For this review, take the finished solid that the model builds, in its own axes (mm). A direction names the side the tool comes from. Give positions to 0.01 mm unless a question says otherwise; leave off trailing zeros. Order: outer loops, then holes, each group sorted by start corner. A loop starts at its lowest first (then second) coordinate and runs counter-clockwise, first axis right, second up. Notation, with made-up numbers: (40.25, -21) -> (93.25, -21) arc R20 ccw to (93.25, 2) -> close; hole circle Ø5 at (-22, -23). An arc over 180 degrees is marked (long way). Return JSON: item names as keys, results as strings. Group by question number.
1) Insertion check: P1, Ø3, axis at x = 2, z = 24, coming from the +Y side; P2, Ø4, axis at x = -14, y = -30.5, coming from the +Z side; P3, Ø12, axis at x = 31.5, y = -22.5, coming from the +Z side; P4, Ø2.5, axis at x = 0, y = 37.5, coming from the +Z side. Each pin has a flat end and moves straight along its axis. Give the tip position at first contact, or say it passes through.
2) For faces 4 (the face through (-14.6, 43.3, 30)), 5 (the face through (2.2, 37.6, 6)), 6 (the face through (-39.717, -19.697, 15.734)), 7 (the face through (42.604, 1.875, 14.434)), 8 (the face through (47, 0, 23)), list the 3-axis set-ups (+Z, -Z, +X, -X, +Y, -Y) from which the entire face can be reached by the end or side of a thin tool; tool diameter is ignored.
3) Add section C-C (x = 0). State how many separate pieces and enclosed holes the cut face has, then the cut area to 3 significant figures.
4) The part is to be moulded in two halves that separate along Y. For faces 1 (the face through (-22.38, -43.028, 14.79)), 2 (the face through (-1, 1, 0)), 3 (the face through (9, 1, 3)), say which applies: released by +Y, released by -Y, zero draft, split by the parting line, or undercut.
5) Add section B-B (y = 0). Give the boundary of the cut face in (x, z).
6) To check wall thickness, follow line 1 along Z through (x, y) = (-46.4, 0); line 2 along Y through (x, z) = (0, 16); line 3 along Y through (x, z) = (0, 6.5). State the ranges of each line that lie inside material, in increasing order.
7) Add section A-A (z = 4.5). Give the boundary of the cut face in (x, y).
from build123d import *

# Parameters (mm, degrees)
F2_R      = 2
F3_DEPTH  = 77.8
F4_R      = 5
F5_DEPTH  = 6
F6_R      = 2
F7_DEPTH  = 12.5
F8_DEPTH  = 12.5
F9_R      = 2
F10_DEPTH = 50
F11_R     = 17.5
F12_DEPTH = 25
F14_R     = 2
F15_DEPTH = 50
F17_R     = 2
F18_DEPTH = 50


with BuildPart() as f1:
    # F0 (on Front) → F1 (revolve)
    with BuildSketch(Plane.XZ):
        Polygon((-48.5, 0), (0, 0), (0, 3), (-45.5, 3), (-45.5, 11.58), (-45.5, 17.58), (-45.5, 30), (-48.5, 30), align=None)
        Polygon((-45.5, 17.58), (-45.5, 11.58), (-42.5, 14.58), (-42.5, 17.58), align=None)
    revolve(axis=Axis((0, 0, 1.5), (0, 0, -1)))

    # F2 (on Front) → F3 (cut, symmetric)
    with BuildSketch(Plane.XZ):
        with Locations((0, 21)):
            Circle(F2_R)
    extrude(amount=F3_DEPTH, both=True, mode=Mode.SUBTRACT)

    # F4 (on Top) → F5 (join)
    with BuildSketch(Plane.XY):
        with Locations((0, -37.5)):
            Circle(F4_R)
        with Locations((0, 37.5)):
            Circle(F4_R)
    extrude(amount=F5_DEPTH)

    # F6 (on face) → F7 (cut, symmetric)
    with BuildSketch(Plane.XY.offset(3)):
        with Locations((0, 37.5)):
            Circle(F6_R)
    extrude(amount=F7_DEPTH, both=True, mode=Mode.SUBTRACT)

    # F6 (on face) → F8 (cut, symmetric)
    with BuildSketch(Plane.XY.offset(3)):
        with Locations((0, -37.5)):
            Circle(F6_R)
    extrude(amount=F8_DEPTH, both=True, mode=Mode.SUBTRACT)

    # F9 (on Right) → F10 (cut, symmetric)
    with BuildSketch(Plane.YZ):
        with Locations((0, 21)):
            Circle(F9_R)
    extrude(amount=F10_DEPTH, both=True, mode=Mode.SUBTRACT)

    # F11 (on face) → F12 (cut, symmetric)
    with BuildSketch(Plane.XY.offset(3)):
        with Locations((-24, -12)):
            Circle(F11_R)
    extrude(amount=F12_DEPTH, both=True, mode=Mode.SUBTRACT)

    # F14 (on face) → F15 (cut, symmetric)
    with BuildSketch(Plane(origin=(0, 0, 0), x_dir=(0.707107, -0.707107, 0), z_dir=(-0.707107, -0.707107, 0))):
        with Locations((0, 21)):
            Circle(F14_R)
    extrude(amount=F15_DEPTH, both=True, mode=Mode.SUBTRACT)

    # F17 (on face) → F18 (cut, symmetric)
    with BuildSketch(Plane(origin=(0, 0, 0), x_dir=(-0.707107, -0.707107, 0), z_dir=(-0.707107, 0.707107, 0))):
        with Locations((0, 21)):
            Circle(F17_R)
    extrude(amount=F18_DEPTH, both=True, mode=Mode.SUBTRACT)


solid = f1.part
Evaluation:
{
 "1": {"P1": "y = 48.5", "P2": "z = 3", "P3": "z = 17.58", "P4": "through"},
 "2": {"face 4": "+Z, +X, -X, +Y, -Y", "face 5": "+Z", "face 6": "+Z, -Z", "face 7": "none", "face 8": "+X, -X"},
 "3": {"separate pieces": "5", "enclosed holes": "0", "area": "468 mm^2"},
 "4": {"face 1": "split by the parting line", "face 2": "zero draft", "face 3": "undercut"},
 "5": {"outline": "(-48.5, 0) -> (-36.74, 0) -> (-36.74, 3) -> (-45.5, 3) -> (-45.5, 11.58) -> (-42.5, 14.58) -> (-42.5, 17.58) -> (-45.5, 17.58) -> (-45.5, 19) -> (-48.5, 19) -> close; (-48.5, 23) -> (-45.5, 23) -> (-45.5, 30) -> (-48.5, 30) -> close; (-11.26, 0) -> (48.5, 0) -> (48.5, 19) -> (45.5, 19) -> (45.5, 17.58) -> (42.5, 17.58) -> (42.5, 14.58) -> (45.5, 11.58) -> (45.5, 3) -> (-11.26, 3) -> close; (45.5, 23) -> (48.5, 23) -> (48.5, 30) -> (45.5, 30) -> close"},
 "6": {"line 1": "0 to 19, 23 to 30", "line 2": "-48.5 to -42.5, 42.5 to 48.5", "line 3": "-48.5 to -45.5, 45.5 to 48.5"},
 "7": {"outline": "circle Ø97 at (0, 0); circle Ø10 at (0, -37.5); circle Ø10 at (0, 37.5); hole circle Ø91 at (0, 0); hole circle Ø4 at (0, -37.5); hole circle Ø4 at (0, 37.5)"}
}
